from build123d import *

# Parameters (mm, degrees)
F0_R      = 3.9
F0_R_2    = 2.4
F1_DEPTH  = 2
F0_R_3    = 5.9
F2_DEPTH  = 2
F4_W      = 15
F4_H      = 15
F5_DEPTH  = 2
F2_FACE_R = 5.9
F5_FACE_W = 15
F5_FACE_H = 15
F8_DEPTH  = 20
F10_DEPTH = 10


with BuildPart() as f1:
    # F0 (on Top) → F1 (new body)
    with BuildSketch(Plane.XY):
        Circle(F0_R)
        Circle(F0_R_2, mode=Mode.SUBTRACT)
        Circle(F0_R_2)
    extrude(amount=F1_DEPTH)

    # F0 (on Top) → F2 (join)
    with BuildSketch(Plane.XY):
        Circle(F0_R_3)
        Circle(F0_R, mode=Mode.SUBTRACT)
    extrude(amount=F2_DEPTH)



with BuildPart() as f5:
    # F4 (on offset) → F5 (new body)
    with BuildSketch(Plane.XY.offset(-5)):
        Rectangle(F4_W, F4_H)
    extrude(amount=-F5_DEPTH)


with BuildPart() as f1_1:
    add(f1.part)

    add(f5.part)  # F6 merges F5
    # F2_face (on face) → F6 section 0
    with BuildSketch(Plane(origin=(0, 0, 0), x_dir=(1, 0, 0), z_dir=(0, 0, -1))):
        Circle(F2_FACE_R)
    # F5_face (on face) → F6 section 1
    with BuildSketch(Plane.XY.offset(-5)):
        Rectangle(F5_FACE_W, F5_FACE_H)
    loft()

    # F7 (on face) → F8 (join)
    with BuildSketch(Plane(origin=(0, 0, -7), x_dir=(1, 0, 0), z_dir=(0, 0, -1))):
        Polygon((-7.5, 1.7), (-7.5, -1.7), (-1.7, -1.7), (-1.7, -7.5), (1.7, -7.5), (1.7, -1.7), (7.5, -1.7), (7.5, 1.7), (1.7, 1.7), (1.7, 7.5), (-1.7, 7.5), (-1.7, 1.7), align=None)
    extrude(amount=F8_DEPTH)

    # F9 (on face) → F10 (cut)
    with BuildSketch(Plane.XY.offset(2)):
        with BuildLine():
            ThreePointArc((1.788854382, -1.1), (2.020716977, -0.5715793024), (2.1, 0))
            ThreePointArc((2.1, 0), (2.020716977, 0.5715793024), (1.788854382, 1.1))
            Line((1.788854382, 1.1), (-1.788854382, 1.1))
            ThreePointArc((-1.788854382, 1.1), (-2.1, 0), (-1.788854382, -1.1))
            Line((-1.788854382, -1.1), (1.788854382, -1.1))
        make_face()
    extrude(amount=-F10_DEPTH, mode=Mode.SUBTRACT)


solid = f1_1.part
Geometry check sheet. Reference: the model listing, model coordinates, mm. A direction names the side the tool comes from. Coordinates: 2 decimals unless noted, no trailing zeros. Order: outer loops, then holes, each group sorted by start corner. A loop starts at its lowest first (then second) coordinate and runs counter-clockwise, first axis right, second up. Notation, with made-up numbers: (-4.5, 8) - (0.5, 8) arc R15 cw to (0.5, 14) - close; hole circle Ø2 at (-12.75, -28). An arc over 180 degrees is marked (long way). Answer in a Markdown table with one row per item. Add a question column.
1) Material ranges on line 1 along X through (y, z) = (-6.25, -14.5); line 2 along Y through (x, z) = (1.5, -1), recorded low to high. Write a range as [from, to].
2) Set-up check for faces 4 (the flat face through (5, -1.7, -17)), 5 (the flat face through (1.7, 5, -17)), 6 (the flat face through (-1.7, 5, -17)), 7 (the flat face through (-5, -5, -7)), 8 (the flat face through (0, 1.1, -3)): record each of +Z, -Z, +X, -X, +Y, -Y from which the full face is reachable in a straight line by a thin tool's end or side.
3) Release check for a two-part mould opening along X. For faces 1 (the flat face through (1.7, -5, -17)), 2 (the cylindrical face through (-2.1, 0, -2.9)), 3 (the flat face through (5, 1.7, -17)) record: +X half, -X half, draft (parallel to the pull), parting line (faces both ways), or undercut.
4) Gauge pin test, flat ends, axial feed: P1, Ø4, axis at y = 4, z = -12.5, coming from the -X side; P2, Ø3, axis at y = -4, z = -14, coming from the +X side; P3, Ø3, axis at x = 4, y = 4, coming from the -Z side. Record the tip position at first contact, or that the pin passes through.
5) Cross-section at A-A, the plane z = -20.5. Record the cut outline in (x, y), then the cut area to 3 significant figures.
Check result:
| question | item | result |
|---|---|---|
| 1 | line 1 | x = [-1.7, 1.7] |
| 1 | line 2 | y = [-6.1, -1.1], [1.1, 6.1] |
| 2 | face 4 | -Z, +X, -Y |
| 2 | face 5 | -Z, +X, +Y |
| 2 | face 6 | -Z, -X, +Y |
| 2 | face 7 | -Z, -X, -Y |
| 2 | face 8 | +Z |
| 3 | face 1 | +X half |
| 3 | face 2 | undercut |
| 3 | face 3 | draft |
| 4 | P1 | stops at x = -1.7 |
| 4 | P2 | stops at x = 1.7 |
| 4 | P3 | stops at z = -7 |
| 5 | outline | (-7.5, -1.7) - (-1.7, -1.7) - (-1.7, -7.5) - (1.7, -7.5) - (1.7, -1.7) - (7.5, -1.7) - (7.5, 1.7) - (1.7, 1.7) - (1.7, 7.5) - (-1.7, 7.5) - (-1.7, 1.7) - (-7.5, 1.7) - close |
| 5 | area | 90.4 mm² |
